```python
from build123d import *

# Parameters (mm, degrees)
ESQUISSE1_R                  = 42.5
BOSS_EXTRU_1_DEPTH           = 6
ENL_V_MAT_EXTRU_6_DEPTH      = 61.402814504
ENL_V_MAT_EXTRU_6_DEPTH_BACK = 6


with BuildPart() as part:
    # Esquisse1 → Boss.-Extru.1 (new body)
    with BuildSketch(Plane.XY):
        Circle(ESQUISSE1_R)
    extrude(amount=BOSS_EXTRU_1_DEPTH)

    # Esquisse3 → Enlèv. mat.-Extru.6 (cut, two sides: drawn at the far end of the back side and taken through both)
    with BuildSketch(Plane.XY.offset(-ENL_V_MAT_EXTRU_6_DEPTH_BACK)):
        with BuildLine():
            Line((-18, -18.9), (18, -18.9))
            ThreePointArc((18, -18.9), (36, -0.9), (18, 17.1))
            Line((18, 17.1), (-18, 17.1))
            ThreePointArc((-18, 17.1), (-36, -0.9), (-18, -18.9))
        make_face()
    extrude(amount=ENL_V_MAT_EXTRU_6_DEPTH + ENL_V_MAT_EXTRU_6_DEPTH_BACK, mode=Mode.SUBTRACT)


solid = part.part
```
Model file for the job. Use its own axes, mm. A direction names the side the tool comes from. Give positions to 0.01 mm unless a question says otherwise; leave off trailing zeros. Write each loop counter-clockwise with the first axis right and the second up, starting at its lowest first coordinate (ties: lowest second). Pieces come first, ordered by that corner, then holes. Notation, with made-up numbers: (-5.5, 6.25) -> (24.5, 6.25) arc R23 cw to (24.5, 32.25) -> close; hole circle Ø6 at (25.25, 48). An arc over 180 degrees is marked (long way). Use CSV: the item, a comma, the result in double quotes. Start each with the question number.
1) Tool access for faces 5 (the cylindrical face through (36, -1, 3)), 6 (the flat face through (-1, 19, 6)): list every direction of +Z, -Z, +X, -X, +Y, -Y with a clear straight run to the whole face (end or side of a thin tool).
2) Cut at C-C on y = 1. List the corners of the cut face in (x, z), plus the area to 3 significant figures.
3) Cut at B-B on x = 0. List the corners of the cut face in (y, z), plus the area to 3 significant figures.
4) Pin check, flat tips, straight feed: P1, Ø3, axis at x = 22.5, y = -17.5, coming from the +Z side; P2, Ø1, axis at y = 32, z = 1.5, coming from the -X side; P3, Ø1.8, axis at x = -8, z = 3.5, coming from the +Y side; P4, Ø2, axis at x = -7, z = 2.5, coming from the +Y side. Stop position of each tip, or through.
5) Two-plate mould, pull along X, no slides. Class faces 1 (the cylindrical face through (-33.727, -25.861, 2.958)), 2 (the flat face through (-1, 19, 0)), 3 (the cylindrical face through (-36, -1, 3)), 4 (the flat face through (0, -18.9, 3)): released by +X, released by -X, zero draft, split by the parting line, or undercut.
6) Cut at A-A on z = 1.5. List the corners of the cut face in (x, y).
7) Drill centre lines: L1, parallel to Y at x = -13.5, z = 1.15; L2, parallel to Y at x = 34.5, z = 1.05; L3, parallel to X at y = 12.5, z = 4.3. Where is each one in solid material? Low to high.
Final values:
1,face 5,"+Z, -Z"
1,face 6,"+Z, +X, -X, +Y, -Y"
2,outline,"(-42.49, 0) -> (-35.9, 0) -> (-35.9, 6) -> (-42.49, 6) -> close; (35.9, 0) -> (42.49, 0) -> (42.49, 6) -> (35.9, 6) -> close"
2,area,"79.1 mm2"
3,outline,"(-42.5, 0) -> (-18.9, 0) -> (-18.9, 6) -> (-42.5, 6) -> close; (17.1, 0) -> (42.5, 0) -> (42.5, 6) -> (17.1, 6) -> close"
3,area,"294 mm2"
4,P1,"stops at z = 6"
4,P2,"stops at x = -28.53"
4,P3,"stops at y = 41.9"
4,P4,"stops at y = 42.07"
5,face 1,"split by the parting line"
5,face 2,"zero draft"
5,face 3,"undercut"
5,face 4,"undercut"
6,outline,"circle Ø85 at (0, 0); hole (-18, -18.9) -> (18, -18.9) arc R18 ccw to (18, 17.1) -> (-18, 17.1) arc R18 ccw to start"
7,L1,"y = -40.3 to -18.9, 17.1 to 40.3"
7,L2,"y = -24.82 to -8.09, 6.29 to 24.82"
7,L3,"x = -40.62 to -30.02, 30.02 to 40.62"
